from build123d import *

# Parameters (mm, degrees)
BOSS_EXTRUDE1_DEPTH = 6
SKETCH2_R           = 1.6
CUT_EXTRUDE1_DEPTH  = 39.547405879


with BuildPart() as part:
    # Sketch1 → Boss-Extrude1 (new body)
    with BuildSketch(Plane.XY):
        with BuildLine():
            Line((-14.535559845, -9.8), (-30, -9.8))
            Line((-30, -9.8), (-30, -5.8))
            Line((-30, -5.8), (-20.459288844, -5.8))
            ThreePointArc((-20.459288844, -5.8), (-18.198720444, -4.772265324), (-17.486995065, -2.393220339))
            ThreePointArc((-17.486995065, -2.393220339), (0, 17.65), (17.486995065, -2.393220339))
            ThreePointArc((17.486995065, -2.393220339), (18.198720444, -4.772265324), (20.459288844, -5.8))
            Line((20.459288844, -5.8), (30, -5.8))
            Line((30, -5.8), (30, -9.8))
            Line((30, -9.8), (14.535559845, -9.8))
            ThreePointArc((14.535559845, -9.8), (11.224237416, -8.043912603), (10.820400779, -4.317571885))
            ThreePointArc((10.820400779, -4.317571885), (0, 11.65), (-10.820400779, -4.317571885))
            ThreePointArc((-10.820400779, -4.317571885), (-11.224237416, -8.043912603), (-14.535559845, -9.8))
        make_face()
    extrude(amount=BOSS_EXTRUDE1_DEPTH)

    # Sketch2 → Cut-Extrude1 (cut, through all)
    with BuildSketch(Plane(origin=(0, -5.8, 0), x_dir=(1, 0, 0), z_dir=(0, 1, 0))):
        with Locations(Location((-25.229644422, -3, 0), (0, 0, 270))):
            Circle(SKETCH2_R)
        with Locations(Location((25.229644422, -3, 0), (0, 0, 90))):
            Circle(SKETCH2_R)
    extrude(amount=-CUT_EXTRUDE1_DEPTH, mode=Mode.SUBTRACT)


solid = part.part
Model file for the job. Use its own axes, mm. A direction names the side the tool comes from. Coordinates: 2 decimals unless noted, no trailing zeros. Write each loop counter-clockwise with the first axis right and the second up, starting at its lowest first coordinate (ties: lowest second). Pieces come first, ordered by that corner, then holes. Notation, with made-up numbers: (-19, 87.25) -> (29, 87.25) arc R27 ccw to (29, 104.25) -> close; hole circle Ø3 at (34, -0.5). An arc over 180 degrees is marked (long way). One line per item, written item: value. Start each with the question number.
1) Slice it at D-D on x = -21. Write the cut outline in (y, z), then the cut area to 3 significant figures.
2) Pull direction Z, two halves, no side cores. Call faces 1 (the face through (-4.3, 11.1, 0)), 2 (the face through (-23.643, -7.772, 2.792)), 3 (the face through (23.643, -7.772, 3.208)), 4 (the face through (11.255, -8.089, 2.958)): +Z half, -Z half, draft (parallel to the pull), parting line (faces both ways), or undercut.
3) Which spindle directions (+Z, -Z, +X, -X, +Y, -Y) get a long thin tool onto all of the face, cutting with end or side? Do faces 5 (the face through (-18.222, -4.799, 2.958)), 6 (the face through (-11.194, -7.998, 2.958)), 7 (the face through (-26.4, -5.8, 1.6)), 8 (the face through (24.1, -5.8, 1.6)). Say none if no direction does.
4) Probe probe 1 along X at (y, z) = (-8.1, 3); probe 2 along X at (y, z) = (-7.75, 3); probe 3 along X at (y, z) = (-0.5, 2.65). List the from-to ranges inside material, lowest first.
5) Flat gauge pins, fed straight in: pin 1 Ø10 at (x, y) = (19.5, 9.5) entering from +Z; pin 2 Ø1 at (y, z) = (10.5, 3.5) entering from +X; pin 3 Ø2 at (y, z) = (-4.5, 3.5) entering from +X; pin 4 Ø2.5 at (x, z) = (-25.23, 3) entering from +Y. Where does each tip first touch, or does it go through?
6) Slice it at C-C on y = 5.75. Write the cut outline in (x, z), then the cut area to 3 significant figures.
7) Slice it at B-B on z = 3. Write the cut outline in (x, y), then the cut area to 3 significant figures.
8) Slice it at A-A on y = 0. Write the cut outline in (x, z).
Answers follow:
1. outline: (-9.8, 0) -> (-5.8, 0) -> (-5.8, 6) -> (-9.8, 6) -> close
1. area: 24.0 mm2
2. face 1: -Z half
2. face 2: undercut
2. face 3: undercut
2. face 4: draft
3. face 5: +Z, -Z, -X
3. face 6: +Z, -Z
3. face 7: +Z, -Z, -X, +Y
3. face 8: +Z, -Z, +X, +Y
4. probe 1: -30 to -26.83, -23.63 to -11.26, 11.26 to 23.63, 26.83 to 30
4. probe 2: -30 to -26.83, -23.63 to -11.04, 11.04 to 23.63, 26.83 to 30
4. probe 3: -17.64 to -11.64, 11.64 to 17.64
5. pin 1: z = 6
5. pin 2: x = 14.54
5. pin 3: x = 19.15
5. pin 4: through
6. outline: (-16.69, 0) -> (-10.13, 0) -> (-10.13, 6) -> (-16.69, 6) -> close; (10.13, 0) -> (16.69, 0) -> (16.69, 6) -> (10.13, 6) -> close
6. area: 78.7 mm2
7. outline: (-30, -9.8) -> (-26.83, -9.8) -> (-26.83, -5.8) -> (-30, -5.8) -> close; (-23.63, -9.8) -> (-14.54, -9.8) arc R4 ccw to (-10.82, -4.32) arc R11.65 cw (long way) to (10.82, -4.32) arc R4 ccw to (14.54, -9.8) -> (23.63, -9.8) -> (23.63, -5.8) -> (20.46, -5.8) arc R3 cw to (17.49, -2.39) arc R17.65 ccw (long way) to (-17.49, -2.39) arc R3 cw to (-20.46, -5.8) -> (-23.63, -5.8) -> close; (26.83, -9.8) -> (30, -9.8) -> (30, -5.8) -> (26.83, -5.8) -> close
7. area: 477 mm2
8. outline: (-17.65, 0) -> (-11.65, 0) -> (-11.65, 6) -> (-17.65, 6) -> close; (11.65, 0) -> (17.65, 0) -> (17.65, 6) -> (11.65, 6) -> close
